from build123d import *

# Parameters (mm, degrees)
SKETCH_1_R          = 12.5
EXTRUDE_1_DEPTH     = 52
SKETCH_2_R          = 3.5
EXTRUDE_2_DEPTH     = 2.5
SKETCH_3_R          = 2
EXTRUDE_3_DEPTH     = 10
CUT_EXTRUDE_1_DEPTH = 10
SKETCH_5_R          = 1.5
CUT_EXTRUDE_2_DEPTH = 7


with BuildPart() as part:
    # 草图1 → 凸台-拉伸1 (new body)
    with BuildSketch(Plane.XY):
        Circle(SKETCH_1_R)
    extrude(amount=EXTRUDE_1_DEPTH)

    # 草图2 → 凸台-拉伸2 (add)
    with BuildSketch(Plane.XY.offset(52)):
        Circle(SKETCH_2_R)
    extrude(amount=EXTRUDE_2_DEPTH)

    # 草图3 → 凸台-拉伸3 (add)
    with BuildSketch(Plane.XY.offset(54.5)):
        Circle(SKETCH_3_R)
    extrude(amount=EXTRUDE_3_DEPTH)

    # 草图4 → 切除-拉伸1 (cut)
    with BuildSketch(Plane.XY.offset(64.5)):
        with BuildLine():
            Line((-0.957908231, -1.755679874), (-0.957908231, 1.755679874))
            ThreePointArc((-0.957908231, 1.755679874), (-2, 0), (-0.957908231, -1.755679874))
        make_face()
    extrude(amount=-CUT_EXTRUDE_1_DEPTH, mode=Mode.SUBTRACT)

    # 草图5 → 切除-拉伸2 (cut)
    with BuildSketch(Plane.XY.offset(52)):
        with Locations((0, 8.5)):
            Circle(SKETCH_5_R)
        with Locations((0, -8.5)):
            Circle(SKETCH_5_R)
    extrude(amount=-CUT_EXTRUDE_2_DEPTH, mode=Mode.SUBTRACT)


solid = part.part
Read the model definition and answer for the solid it produces. Units are mm, in the model's axes. A direction names the side the tool comes from. Round coordinates to 2 decimals unless told otherwise and drop trailing zeros. Write each loop counter-clockwise with the first axis right and the second up, starting at its lowest first coordinate (ties: lowest second). Pieces come first, ordered by that corner, then holes. Notation, with made-up numbers: (-18.75, 65) - (38.25, 65) arc R22 ccw to (38.25, 87) - close; hole circle Ø2 at (-38.75, 16). An arc over 180 degrees is marked (long way). One line per question, with ' | ' between items. Start each with the question number.
1. Each of these flat-tipped pins is pushed along its axis until it touches: pin 1 (2 mm diameter, centred on y = 0.5, z = 57, fed in from -X); pin 2 (1 mm diameter, centred on x = 7.5, y = -1, fed in from +Z); pin 3 (1 mm diameter, centred on x = -1.5, z = 23, fed in from -Y). Where does it stop, or does it pass through?
2. Section D-D (y = -8.5) is taken. Determine the outline of the cut face in (x, z), and give its area (3 significant figures).
3. For faces 1 (the face through (-0.958, 0, 60)), 2 (the face through (11.923, 3.755, 25.636)), 3 (the face through (3, -3, 52)), determine the directions among +Z, -Z, +X, -X, +Y, -Y from which every point of the face is accessible in a straight line to the end or side of a thin tool.
4. Find the intervals of material crossed by probe 1 along Y at (x, z) = (0, 48); probe 2 along Z at (x, y) = (-0.5, -10); probe 3 along Z at (x, y) = (0, 2.25), in increasing order. Write a range as [from, to].
5. Section C-C (z = 60) is taken. Determine the outline of the cut face in (x, y), and give its area (3 significant figures).
6. Section B-B (x = 0) is taken. Determine the outline of the cut face in (y, z).
7. For a pull along Y with two mould halves and no side action, classify faces 4 (the face through (0, 7, 49)), 5 (the face through (3.233, -1.341, 53.232)), 6 (the face through (0, -8, 45)), 7 (the face through (-2, 0, 54.5)) as +Y half, -Y half, draft (parallel to the pull), parting line (faces both ways), or undercut.
8. Section A-A (y = 0) is taken. Determine the outline of the cut face in (x, z), and give its area (3 significant figures).
Filled in:
1) pin 1: x = -0.96 | pin 2: z = 52 | pin 3: y = -12.46
2) outline: (-9.17, 0) - (9.17, 0) - (9.17, 52) - (1.5, 52) - (1.5, 45) - (-1.5, 45) - (-1.5, 52) - (-9.17, 52) - close | area: 932 mm²
3) face 1: +Z, -X, +Y, -Y | face 2: +Z, -Z | face 3: +Z
4) probe 1: [-12.5, -10], [-7, 7], [10, 12.5] | probe 2: [0, 52] | probe 3: [0, 54.5]
5) outline: (-0.96, -1.76) arc R2 ccw (long way) to (-0.96, 1.76) - close | area: 9.96 mm²
6) outline: (-12.5, 0) - (12.5, 0) - (12.5, 52) - (10, 52) - (10, 45) - (7, 45) - (7, 52) - (3.5, 52) - (3.5, 54.5) - (2, 54.5) - (2, 64.5) - (-2, 64.5) - (-2, 54.5) - (-3.5, 54.5) - (-3.5, 52) - (-7, 52) - (-7, 45) - (-10, 45) - (-10, 52) - (-12.5, 52) - close
7) face 4: undercut | face 5: parting line | face 6: undercut | face 7: draft
8) outline: (-12.5, 0) - (12.5, 0) - (12.5, 52) - (3.5, 52) - (3.5, 54.5) - (2, 54.5) - (2, 64.5) - (-0.96, 64.5) - (-0.96, 54.5) - (-3.5, 54.5) - (-3.5, 52) - (-12.5, 52) - close | area: 1,350 mm²
